```python
from build123d import *

# Parameters (mm, degrees)
BOSS_EXTRUDE1_DEPTH = 10
SKETCH2_R           = 3.25
SKETCH2_W           = 20
SKETCH2_H           = 37
CUT_EXTRUDE1_DEPTH  = 10
CUT_EXTRUDE2_START  = -3
SKETCH3_W           = 20
SKETCH3_H           = 37
SKETCH3_R           = 3.25
CUT_EXTRUDE2_DEPTH  = 3
FILLET1_R           = 5
CUT_EXTRUDE3_DEPTH  = 3
SKETCH5_R           = 2.5
CUT_EXTRUDE4_DEPTH  = 7


with BuildPart() as part:
    # Sketch1 → Boss-Extrude1 (new body)
    with BuildSketch(Plane.XY):
        with BuildLine():
            Line((-72.324772809, -75.56835732), (113.0098159, -145.404579152))
            ThreePointArc((113.0098159, -145.404579152), (122.225331612, -144.27064673), (126.535908242, -136.046872553))
            Line((126.535908242, -136.046872553), (126.535908242, 37.498632429))
            ThreePointArc((126.535908242, 37.498632429), (123.606976053, 44.569700241), (116.535908242, 47.498632429))
            Line((116.535908242, 47.498632429), (-45.464091758, 47.498632429))
            ThreePointArc((-45.464091758, 47.498632429), (-51.711042234, 45.307320523), (-55.220189319, 39.69375438))
            Line((-55.220189319, 39.69375438), (-78.554778028, -64.01552877))
            ThreePointArc((-78.554778028, -64.01552877), (-77.600447564, -70.957112136), (-72.324772809, -75.56835732))
        make_face()
    extrude(amount=BOSS_EXTRUDE1_DEPTH)

    # Sketch2 → Cut-Extrude1 (cut)
    with BuildSketch(Plane.XY.offset(10)):
        with Locations((43.734834886, 17.498632429)):
            Circle(SKETCH2_R)
        with Locations((96.535908242, -1.501367571)):
            Circle(SKETCH2_R)
        with Locations((96.535908242, -47.501367571)):
            Circle(SKETCH2_R)
        with Locations((96.535908242, -98.501367571)):
            Circle(SKETCH2_R)
        with Locations((46.535908242, -57.501367571)):
            Circle(SKETCH2_R)
        with Locations((46.535908242, -99.501367571)):
            Circle(SKETCH2_R)
        with Locations((-16.798680467, -51.001367571)):
            Rectangle(SKETCH2_W, SKETCH2_H)
        Polygon((-30.265165114, 40.498632429), (19.734834886, 40.498632429), (25.734834886, 34.498632429), (25.734834886, -7.501367571), (19.734834886, -13.501367571), (-30.265165114, -13.501367571), (-36.265165114, -7.501367571), (-36.265165114, 34.498632429), align=None)
    extrude(amount=-CUT_EXTRUDE1_DEPTH, mode=Mode.SUBTRACT)

    # Sketch3 → Cut-Extrude2 (cut)
    with BuildSketch(Plane.XY.offset(10).offset(CUT_EXTRUDE2_START)):
        with BuildLine():
            Line((-72.324772809, -75.56835732), (-2.464091758, -101.892671919))
            Line((-2.464091758, -101.892671919), (-2.464091758, -29.501367571))
            ThreePointArc((-2.464091758, -29.501367571), (-0.413839227, -24.551620103), (4.535908242, -22.501367571))
            Line((4.535908242, -22.501367571), (30.105771034, -22.501367571))
            ThreePointArc((30.105771034, -22.501367571), (32.401500165, -22.114205672), (34.443281054, -20.99554693))
            Line((34.443281054, -20.99554693), (49.628535429, -9.007188212))
            ThreePointArc((49.628535429, -9.007188212), (51.670316318, -7.88852947), (53.966045449, -7.501367571))
            Line((53.966045449, -7.501367571), (60.535908242, -7.501367571))
            ThreePointArc((60.535908242, -7.501367571), (65.48565571, -5.451115039), (67.535908242, -0.501367571))
            Line((67.535908242, -0.501367571), (67.535908242, 47.498632429))
            Line((67.535908242, 47.498632429), (-45.464091733, 47.498632429))
            ThreePointArc((-45.464091733, 47.498632429), (-51.710766684, 45.307540935), (-55.220034365, 39.69444284))
            Line((-55.220034365, 39.69444284), (-55.220189319, 39.69375438))
            Line((-55.220189319, 39.69375438), (-78.554778028, -64.01552877))
            ThreePointArc((-78.554778028, -64.01552877), (-77.600447564, -70.957112136), (-72.324772809, -75.56835732))
        make_face()
        with Locations((-16.798680467, -51.001367571)):
            Rectangle(SKETCH3_W, SKETCH3_H, mode=Mode.SUBTRACT)
        Polygon((-30.265165114, -13.501367571), (-36.265165114, -7.501367571), (-36.265165114, 34.498632429), (-30.265165114, 40.498632429), (19.734834886, 40.498632429), (25.734834886, 34.498632429), (25.734834886, -7.501367571), (19.734834886, -13.501367571), align=None, mode=Mode.SUBTRACT)
        with Locations((43.734834886, 17.498632429)):
            Circle(SKETCH3_R, mode=Mode.SUBTRACT)
    extrude(amount=CUT_EXTRUDE2_DEPTH, mode=Mode.SUBTRACT)

    # Fillet1
    fillet1_edges = [part.edges().sort_by_distance(p)[0] for p in [
        (-2.464091758, -101.892671919, 8.5),
        (67.535908242, 47.498632429, 8.5),
    ]]
    fillet(fillet1_edges, radius=FILLET1_R)

    # Sketch4 → Cut-Extrude3 (cut)
    with BuildSketch(Plane.XY.offset(10)):
        with BuildLine():
            Line((126.535908242, 22.498632429), (118.535908242, 22.498632429))
            ThreePointArc((118.535908242, 22.498632429), (115.000374336, 23.963098523), (113.535908242, 27.498632429))
            Line((113.535908242, 27.498632429), (113.535908242, 47.498632429))
            Line((113.535908242, 47.498632429), (126.535908242, 47.498632429))
            Line((126.535908242, 47.498632429), (126.535908242, 22.498632429))
        make_face()
        with BuildLine():
            Line((126.535908242, -123.046872553), (119.535908242, -123.046872553))
            ThreePointArc((119.535908242, -123.046872553), (116.000374336, -124.511338647), (114.535908242, -128.046872553))
            Line((114.535908242, -128.046872553), (114.535908242, -146.046872553))
            Line((114.535908242, -146.046872553), (126.535908242, -146.046872553))
            Line((126.535908242, -146.046872553), (126.535908242, -123.046872553))
        make_face()
    extrude(amount=-CUT_EXTRUDE3_DEPTH, mode=Mode.SUBTRACT)

    # Sketch5 → Cut-Extrude4 (cut)
    with BuildSketch(Plane.XY.offset(7)):
        with Locations((120.535908242, -129.046872553)):
            Circle(SKETCH5_R)
        with Locations((119.535908242, 28.498632429)):
            Circle(SKETCH5_R)
        with Locations((-47.220189319, 39.498632429)):
            Circle(SKETCH5_R)
        with Locations((-70.554778028, -67.56835732)):
            Circle(SKETCH5_R)
    extrude(amount=-CUT_EXTRUDE4_DEPTH, mode=Mode.SUBTRACT)


solid = part.part
```
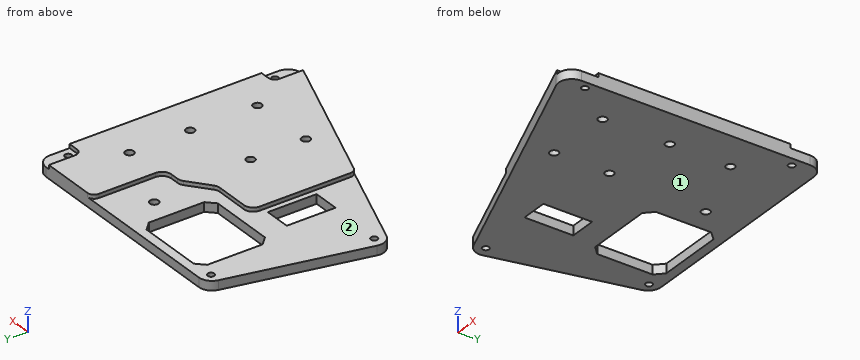
Read the model definition and answer for the solid it produces. Units are mm, in the model's axes. Face numbers are marked on the shaded views. A direction names the side the tool comes from. Coordinates: 2 decimals unless noted, no trailing zeros. Write each loop counter-clockwise with the first axis right and the second up, starting at its lowest first coordinate (ties: lowest second). Pieces come first, ordered by that corner, then holes. Notation, with made-up numbers: (2.5, -37.5) -> (24.5, -37.5) arc R20 ccw to (24.5, -6.5) -> close; hole circle Ø9 at (50.5, 83). An arc over 180 degrees is marked (long way). Return JSON: item names as keys, results as strings.
1. A cutting plane is placed at A-A (x = 9). Determine the outline of the cut face in (y, z), and give its area (3 significant figures).
Found:
{"outline": "(-106.21, 0) -> (-13.5, 0) -> (-13.5, 7) -> (-22.5, 7) -> (-22.5, 10) -> (-106.21, 10) -> close; (40.5, 0) -> (47.5, 0) -> (47.5, 7) -> (40.5, 7) -> close", "area": "949 mm2"}
2. A cutting plane is placed at D-D (x = -42). Determine the outline of the cut face in (y, z), and give its area (3 significant figures).
Found:
{"outline": "(-87, 0) -> (47.5, 0) -> (47.5, 7) -> (-87, 7) -> close", "area": "941 mm2"}
3. Find the intervals of material crossed by line 1 along X through (y, z) = (19.5, 2.25); line 2 along Y through (x, z) = (-14.5, 2.25); line 3 along X through (y, z) = (-59, 5.5), in increasing order. Write a range as from..to.
Found:
{"line 1": "-59.76..-36.27, 25.73..41.17, 46.3..126.54", "line 2": "-97.36..-69.5, -32.5..-13.5, 40.5..47.5", "line 3": "-77.43..-26.8, -6.8..43.65, 49.42..126.54"}
4. A cutting plane is placed at B-B (z = 3). Give the number of separate pieces and of enclosed holes in the cut face, and give its area (3 significant figures).
Found:
{"separate pieces": "1", "enclosed holes": "12", "area": "26,900 mm2"}
5. A cutting plane is placed at C-C (y = -90). Determine the outline of the cut face in (x, z).
Found:
{"outline": "(-34.03, 0) -> (126.54, 0) -> (126.54, 10) -> (-2.46, 10) -> (-2.46, 7) -> (-34.03, 7) -> close"}
6. Each of these flat-tipped pins is pushed along its axis until it touches: P1, Ø8.5, axis at x = 43.73, y = 17.5, coming from the +Z side; P2, Ø2.5, axis at y = 20.5, z = 8, coming from the -X side; P3, Ø3, axis at x = -47.22, y = 39.5, coming from the +Z side; P4, Ø3.5, axis at y = -57, z = 9, coming from the -X side. Where does it stop, or does it pass through?
Found:
{"P1": "z = 7", "P2": "x = -59.71", "P3": "through", "P4": "x = -2.46"}
7. A tool of negligible diameter and unlimited length cuts with its end or side. For the marked faces 1 and 2, from which of +Z, -Z, +X, -X, +Y, -Y can it reach the whole face along a straight path? Write none if from no direction.
Found:
{"face 1": "-Z, +X, -X, +Y, -Y", "face 2": "+Z, -X, +Y"}
